Here's how the part is built. I have some questions about the finished solid (model axes, mm). Coordinates: 2 decimals unless noted, no trailing zeros. Write each loop counter-clockwise with the first axis right and the second up, starting at its lowest first coordinate (ties: lowest second). Pieces come first, ordered by that corner, then holes. Notation, with made-up numbers: (11.5, -10) -> (64.5, -10) arc R18 ccw to (64.5, 0) -> close; hole circle Ø3 at (8, -3). An arc over 180 degrees is marked (long way). Use CSV: the item, a comma, the result in double quotes. Start each with the question number.
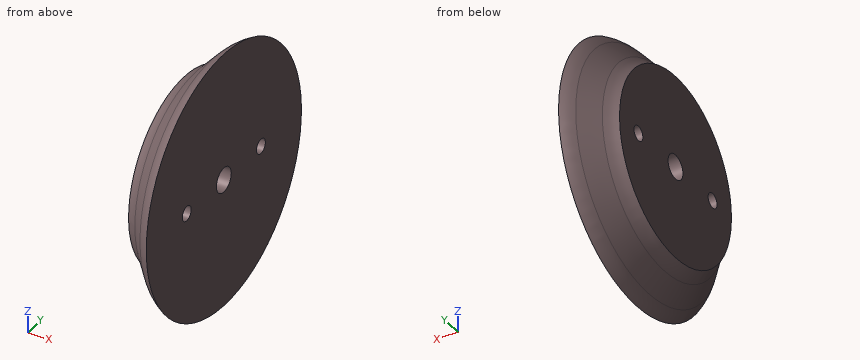
Autodesk Inventor part; units mm, degrees
ref_plane "YZ Plane" through (0, 0, 0) normal (1, 0, 0) x (0, 1, 0)
ref_plane "XZ Plane" through (0, 0, 0) normal (0, 1, 0) x (-1, 0, 0)
ref_plane "XY Plane" through (0, 0, 0) normal (0, 0, 1) x (1, 0, 0)
sketch "Sketch1" plane through (0, 0, 0) normal (0, 1, 0) x (-1, 0, 0)
  line L0 (0, 0) -> (0, -18) construction
  line L1 (0, 0) -> (-8, 0)
  line L2 (-8, 0) -> (-8, -27) construction
  line L3 (-2.3867, -20.6851) -> (-5.6133, -24.3149)
  arc A0 (0, -18.852) -> (-2.3867, -20.6851) centre (3.5925, -26) ccw
  arc A1 (-8, -26.148) -> (-5.6133, -24.3149) centre (-11.5925, -19) ccw
  line L4 (0, 0) -> (0, -18.852)
  line L5 (-8, 0) -> (-8, -26.148)
  dimension "d0" = 18
  dimension "d1" = 8
  dimension "d2" = 27
  dimension "d3" = 8
revolve "Revolution1" add sketch "Sketch1" angle 360 about axis through (0, 0, 0) along (1, 0, 0)
sketch "Sketch2" plane through (0, 0, 0) normal (-1, 0, 0) x (0, 0, 1)
  circle A0 centre (0, 0) radius 2.5
  line L0 (0, 0) -> (0, 12.5) construction
  circle A1 centre (0, 12.5) radius 1.5
  line L1 (0, 0) -> (0, -12.5) construction
  circle A2 centre (0, -12.5) radius 1.5
  dimension "d5" = 5
  dimension "d6" = 12.5
  dimension "d7" = 12.5
  dimension "d8" = 3
  dimension "d9" = 3
extrude "Extrusion1" cut sketch "Sketch2" against normal blind 10
properties part number "gearboxmotorconnection"
Item 1: I want a section at C-C on x = 3.25. Please give me the cut outline in (y, z).
Item 2: I want a section at B-B on y = 0. Please give me the cut outline in (x, z), then the cut area to 3 significant figures.
Item 3: I want a section at A-A on z = 0. Please give me the cut outline in (x, y), then the cut area to 3 significant figures.
Item 4: I'm going to push flat-ended pins straight in: pin 1 (10 mm diameter, centred on y = -11.5, z = -20, fed in from -X); pin 2 (1.5 mm diameter, centred on x = 4.5, z = -12.5, fed in from +Y); pin 3 (1 mm diameter, centred on x = 3, z = -4.5, fed in from -Y); pin 4 (3 mm diameter, centred on x = 3.5, y = 12.5, fed in from -Z). Where does each tip first touch, or does it pass through?
Item 5: If I drill on line 1 along Y through (x, z) = (5.75, 0); line 2 along Y through (x, z) = (2.25, 0); line 3 along Z through (x, y) = (5, -11.5), over which ranges is the centre line in solid material (lowest first)?
Geometry says:
1,outline,"circle Ø43.31 at (0, 0); hole circle Ø3 at (-12.5, 0); hole circle Ø5 at (0, 0); hole circle Ø3 at (12.5, 0)"
2,outline,"(0, -18.85) arc R8 cw to (2.39, -20.69) -> (5.61, -24.31) arc R8 ccw to (8, -26.15) -> (8, -2.5) -> (0, -2.5) -> close; (0, 2.5) -> (8, 2.5) -> (8, 26.15) arc R8 ccw to (5.61, 24.31) -> (2.39, 20.69) arc R8 cw to (0, 18.85) -> close"
2,area,"320 mm2"
3,outline,"(0, -18.85) arc R8 cw to (2.39, -20.69) -> (5.61, -24.31) arc R8 ccw to (8, -26.15) -> (8, -14) -> (0, -14) -> close; (0, -11) -> (8, -11) -> (8, -2.5) -> (0, -2.5) -> close; (0, 2.5) -> (8, 2.5) -> (8, 11) -> (0, 11) -> close; (0, 14) -> (8, 14) -> (8, 26.15) arc R8 ccw to (5.61, 24.31) -> (2.39, 20.69) arc R8 cw to (0, 18.85) -> close"
3,area,"272 mm2"
4,pin 1,"x = 0"
4,pin 2,"y = 20.48"
4,pin 3,"y = -21.48"
4,pin 4,"z = -20.25"
5,line 1,"-24.46 to -14, -11 to -2.5, 2.5 to 11, 14 to 24.46"
5,line 2,"-20.54 to -14, -11 to -2.5, 2.5 to 11, 14 to 20.54"
5,line 3,"-20.64 to -1.12, 1.12 to 20.64"
